For this review, take the finished solid that the model builds, in its own axes (mm). A direction names the side the tool comes from. Coordinates: 2 decimals unless noted, no trailing zeros. Write each loop counter-clockwise with the first axis right and the second up, starting at its lowest first coordinate (ties: lowest second). Pieces come first, ordered by that corner, then holes. Notation, with made-up numbers: (60.5, 34) -> (87.5, 34) arc R16 ccw to (87.5, 53) -> close; hole circle Ø8 at (-39, -33.5). An arc over 180 degrees is marked (long way). One line per item, written item: value. Start each with the question number.
1) Add section B-B (z = -3.5). State the section outline as (x, y) points, and give its area (3 significant figures).
2) Machinability: for faces 1 (the flat face through (-9, -25.4, 0)), 2 (the flat face through (27, -25.4, 0)), 3 (the flat face through (-9, 25.4, 0)), 4 (the flat face through (0, -27, 0)), 5 (the flat face through (27, 25.4, 0)), which of the approach directions +Z, -Z, +X, -X, +Y, -Y give a long, thin tool a straight path to every point of the face, cutting with its end or side? Answer none if there is none.
3) Add section A-A (x = 1). State the section outline as (y, z) points, and give its area (3 significant figures).
4) Add section C-C (y = -8). State the section outline as (x, z) points.
5) For probe 1 along Y at (x, z) = (-10, -4.5); probe 2 along X at (y, z) = (-26, -15); probe 3 along X at (y, z) = (-19.5, -1.5), list the stretches that pass through material, from the lowest coordinate up. Write a range as from..to.
6) Add section D-D (z = -23). State the section outline as (x, y) points, and give its area (3 significant figures).
7) For pin 1 Ø1.5 at (y, z) = (15.5, 1) entering from +X; pin 2 Ø3 at (x, y) = (-15, 13) entering from -Z; pin 3 Ø10 at (x, z) = (1.5, 7) entering from -Y, all flat-tipped, find the tip position at first contact; note any pin that passes through.
from build123d import *

# Parameters (mm, degrees)
F0_R      = 30.41715
F2_DEPTH  = 25.4
F2_FACE_R = 30.41715
F3_DEPTH  = 25.4
F1_R      = 30.664626
F4_DEPTH  = 25.4


with BuildPart() as f2:
    # F0 (on Front) → F2 (new body)
    with BuildSketch(Plane.XZ):
        Circle(F0_R)
    extrude(amount=F2_DEPTH)

    # F2_face (on face) → F3 (join)
    with BuildSketch(Plane(origin=(0, 0, 0), x_dir=(1, 0, 0), z_dir=(0, 1, 0))):
        Circle(F2_FACE_R)
    extrude(amount=F3_DEPTH)

    # F1 (on Right) → F4 (join)
    with BuildSketch(Plane.YZ):
        with Locations((0.104457, -0.068773)):
            Circle(F1_R)
    extrude(amount=F4_DEPTH)


solid = f2.part
Numbers:
1. outline: (-30.22, -25.4) -> (0, -25.4) -> (0, -30.37) -> (25.4, -30.37) -> (25.4, -25.4) -> (30.22, -25.4) -> (30.22, 25.4) -> (25.4, 25.4) -> (25.4, 30.58) -> (0, 30.58) -> (0, 25.4) -> (-30.22, 25.4) -> close
1. area: 3,330 mm²
2. face 1: -X, -Y
2. face 2: +Z, -Z, +X, -Y
2. face 3: -X, +Y
2. face 4: +Z, -Z, -X, -Y
2. face 5: +Z, -Z, +X, +Y
3. outline: (-25.4, -30.4) -> (-4.4, -30.4) arc R30.66 ccw to (4.61, -30.4) -> (25.4, -30.4) -> (25.4, -17.4) arc R30.66 ccw to (25.4, 17.26) -> (25.4, 30.4) -> (3.56, 30.4) arc R30.66 ccw to (-3.35, 30.4) -> (-25.4, 30.4) -> (-25.4, 16.96) arc R30.66 ccw to (-25.4, -17.09) -> close
3. area: 3,340 mm²
4. outline: (6.82, -29.64) -> (25.4, -29.64) -> (25.4, -16.73) arc R30.42 ccw to (25.4, 16.73) -> (25.4, 29.51) -> (7.39, 29.51) arc R30.42 ccw (long way) to start
5. probe 1: -25.4..25.4
5. probe 2: 0..25.4
5. probe 3: -30.38..30.38
6. outline: (-19.9, -25.4) -> (19.9, -25.4) -> (19.9, -20.25) -> (25.4, -20.25) -> (25.4, 20.46) -> (19.9, 20.46) -> (19.9, 25.4) -> (-19.9, 25.4) -> close
6. area: 2,250 mm²
7. pin 1: x = 30.42
7. pin 2: z = -27.26
7. pin 3: y = -30.49
